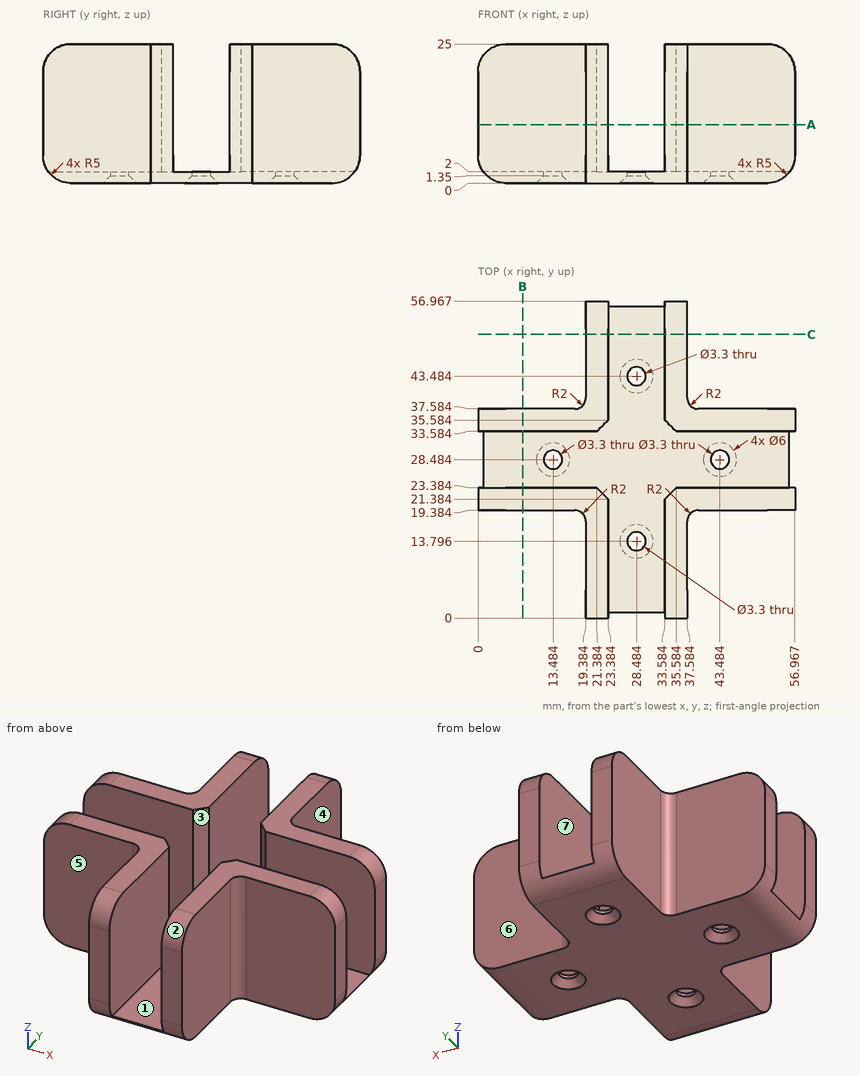
Could you check a few things on this drawing? It's one solid part, dimensions in mm from its lowest x, y, z. A direction names the side the tool comes from. Coordinates: 2 decimals unless noted, no trailing zeros. Order: outer loops, then holes, each group sorted by start corner. A loop starts at its lowest first (then second) coordinate and runs counter-clockwise, first axis right, second up. Notation, with made-up numbers: (43.5, -37.75) -> (53.5, -37.75) arc R23 ccw to (53.5, -25.75) -> close; hole circle Ø7 at (36.25, 85.25). An arc over 180 degrees is marked (long way). One line per item, written item: value. Start each with the question number.
1) Imagine slicing it at B-B on x = 8. List the corners of the cut face in (y, z) for me, plus the area to 3 significant figures.
2) If I drill on L1, parallel to Y at x = 15, z = 2.25; L2, parallel to Z at x = 6, y = 31.5, over which ranges is the centre line in solid material (lowest first)? Write a range as [from, to].
3) Which directions (+Z, -Z, +X, -X, +Y, -Y) give clear straight access to the entire face, cutting with the end or side of a thin tool? Please do the marked faces 5, 6 and 7.
4) Imagine slicing it at A-A on z = 10.5. Count the separate pieces of the cut face and the enclosed holes in it.
5) We'd pull the mould along Y, two halves only. Please class the marked faces 1, 2, 3 and 4: +Y half, -Y half, draft (parallel to the pull), parting line (faces both ways), or undercut.
6) I'm going to push flat-ended pins straight in: pin 1 (5 mm diameter, centred on x = 9.5, z = 10, fed in from +Y); pin 2 (4 mm diameter, centred on x = 20, z = 4.5, fed in from +Y); pin 3 (2 mm diameter, centred on y = 46.5, z = 8, fed in from +X); pin 4 (8.5 mm diameter, centred on x = 44, z = 13, fed in from -Y). Where does each tip first touch, or does it pass through?
Answer list:
1. outline: (19.38, 0) -> (37.58, 0) -> (37.58, 25) -> (33.58, 25) -> (33.58, 2) -> (23.38, 2) -> (23.38, 25) -> (19.38, 25) -> close
1. area: 220 mm2
2. L1: y = [19.38, 23.38], [33.58, 37.58]
2. L2: z = [0, 2]
3. face 5: +Z, -Z, -X, -Y
3. face 6: +Z, -Z, +X, +Y
3. face 7: +Z, +Y, -Y
4. separate pieces: 4
4. enclosed holes: 0
5. face 1: undercut
5. face 2: -Y half
5. face 3: undercut
5. face 4: draft
6. pin 1: stops at y = 37.58
6. pin 2: stops at y = 56.97
6. pin 3: stops at x = 37.58
6. pin 4: stops at y = 19.38
